The model under review builds one solid part; all positions refer to its coordinate system, in mm. A direction names the side the tool comes from. Give positions to 0.01 mm unless a question says otherwise; leave off trailing zeros. Order: outer loops, then holes, each group sorted by start corner. A loop starts at its lowest first (then second) coordinate and runs counter-clockwise, first axis right, second up. Notation, with made-up numbers: (-20.5, 60.25) -> (-9.5, 60.25) arc R21 ccw to (-9.5, 74.25) -> close; hole circle Ø9 at (81, -16.75). An arc over 180 degrees is marked (long way). Answer as a JSON object with one key per item and string values. Group by question number.
from build123d import *

# Parameters (mm, degrees)
SKETCH1_W           = 120.7
SKETCH1_H           = 75.8
BOSS_EXTRUDE1_DEPTH = 4.2
SKETCH2_W           = 48.4
SKETCH2_H           = 47.4
BOSS_EXTRUDE2_DEPTH = 0.3
SKETCH4_W           = 27.08
SKETCH4_H           = 22.41
CUT_EXTRUDE1_DEPTH  = 0.3
FILLET2_R           = 1
FILLET3_R           = 2


with BuildPart() as part:
    # Sketch1 → Boss-Extrude1 (new body)
    with BuildSketch(Plane(origin=(0, 0, 0), x_dir=(1, 0, 0), z_dir=(0, 1, 0))):
        with Locations((60.35, -37.9)):
            Rectangle(SKETCH1_W, SKETCH1_H)
    extrude(amount=BOSS_EXTRUDE1_DEPTH)

    # Sketch2 → Boss-Extrude2 (add)
    with BuildSketch(Plane(origin=(0, 4.2, 0), x_dir=(1, 0, 0), z_dir=(0, 1, 0))):
        with Locations((70.5, -99.5)):
            Rectangle(SKETCH2_W, SKETCH2_H)
    extrude(amount=-BOSS_EXTRUDE2_DEPTH)

    # Sketch4 → Cut-Extrude1 (cut)
    with BuildSketch(Plane.XZ.offset(-3.9)):
        with Locations((59.84, 111.995)):
            Rectangle(SKETCH4_W, SKETCH4_H)
    extrude(amount=-CUT_EXTRUDE1_DEPTH, mode=Mode.SUBTRACT)

    # Fillet2
    fillet2_edges = [part.edges().sort_by_distance(p)[0] for p in [
        (94.7, 4.05, 123.2),
        (46.3, 4.05, 100.79),
        (73.38, 4.05, 123.2),
        (73.38, 4.05, 100.79),
    ]]
    fillet(fillet2_edges, radius=FILLET2_R)

    # Fillet3
    fillet3_edges = [part.edges().sort_by_distance(p)[0] for p in [
        (0, 2.1, 0),
        (120.7, 2.1, 0),
        (120.7, 2.1, 75.8),
        (0, 2.1, 75.8),
    ]]
    fillet(fillet3_edges, radius=FILLET3_R)


solid = part.part
1. Take a section at B-B on y = 2.5. Give the boundary of the cut face in (x, z).
2. Machinability: for faces 1 (the flat face through (0, 2, 38)), 2 (the flat face through (76, 3.9, 94)), which of the approach directions +Z, -Z, +X, -X, +Y, -Y give a long, thin tool a straight path to every point of the face, cutting with its end or side? Answer none if there is none.
3. For probe 1 along Z at (x, y) = (25, 0.8); probe 2 along Y at (x, z) = (67, 84.5), list the stretches that pass through material, from the lowest coordinate up. Write a range as [from, to].
4. Take a section at C-C on z = 92.5. Give the boundary of the cut face in (x, y), plus the area to 3 significant figures.
5. For pin 1 (1.5 mm diameter, centred on x = 104, y = 3.5, fed in from +Z); pin 2 (4 mm diameter, centred on x = 23, z = 20.5, fed in from -Y); pin 3 (23.5 mm diameter, centred on x = 75.5, z = 90.5, fed in from -Y), all flat-tipped, find the tip position at first contact; note any pin that passes through.
6. Take a section at A-A on x = 58. Give the boundary of the cut face in (y, z).
7. Take a section at D-D on x = 85. Give the boundary of the cut face in (y, z).
Checks:
{
 "1": {"outline": "(0, 2) arc R2 ccw to (2, 0) -> (118.7, 0) arc R2 ccw to (120.7, 2) -> (120.7, 73.8) arc R2 ccw to (118.7, 75.8) -> (2, 75.8) arc R2 ccw to (0, 73.8) -> close"},
 "2": {"face 1": "+Z, -Z, -X, +Y, -Y", "face 2": "+Z, +X, -X, -Y"},
 "3": {"probe 1": "z = [0, 75.8]", "probe 2": "y = [3.9, 4.2]"},
 "4": {"outline": "(46.3, 3.9) -> (94.7, 3.9) -> (94.7, 4.2) -> (46.3, 4.2) -> close", "area": "14.5 mm2"},
 "5": {"pin 1": "stops at z = 75.8", "pin 2": "stops at y = 0", "pin 3": "stops at y = 3.9"},
 "6": {"outline": "(0, 0) -> (4.2, 0) -> (4.2, 100.79) -> (3.9, 100.79) -> (3.9, 75.8) -> (0, 75.8) -> close"},
 "7": {"outline": "(0, 0) -> (4.2, 0) -> (4.2, 123.2) -> (3.9, 123.2) -> (3.9, 75.8) -> (0, 75.8) -> close"}
}
